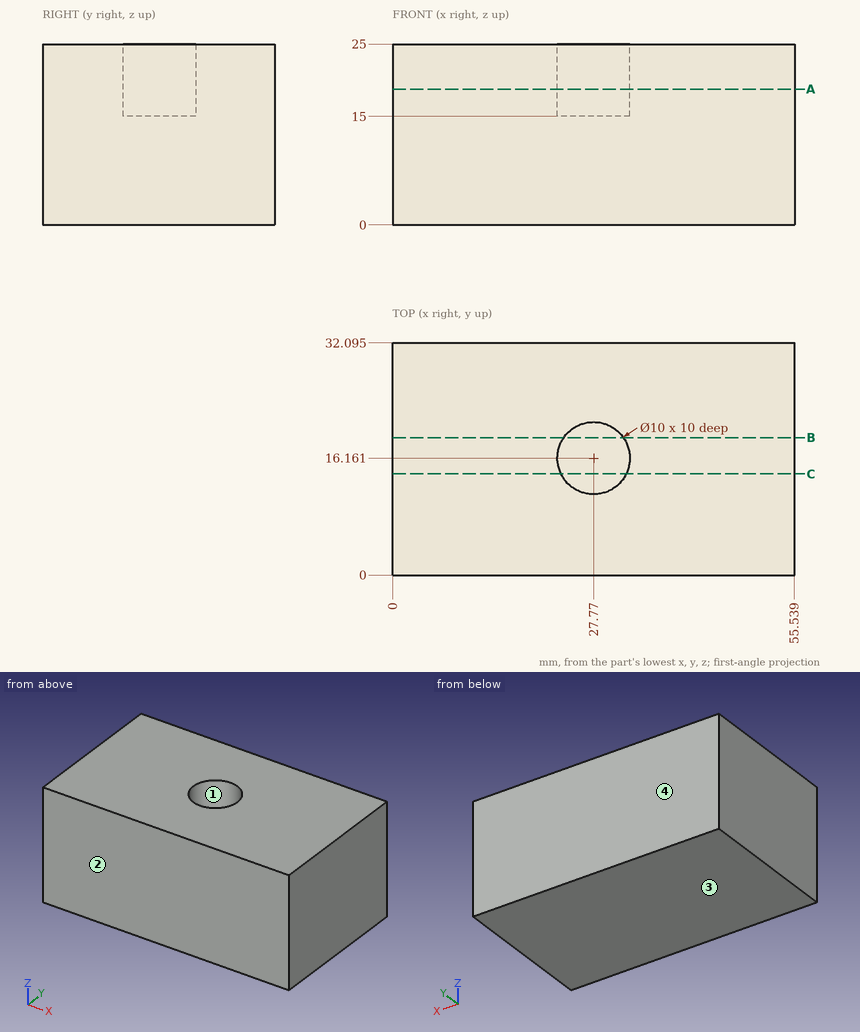
Input: dimensioned drawing with shaded views. Units: mm. Origin: part minimum x, y, z. Coordinates: 2 decimals unless noted, no trailing zeros. Order: outer loops, then holes, each group sorted by start corner. A loop starts at its lowest first (then second) coordinate and runs counter-clockwise, first axis right, second up. Notation, with made-up numbers: (9.25, 15.25) - (43.25, 15.25) arc R35 cw to (43.25, 52.25) - close; hole circle Ø5 at (-22.5, 1.25). An arc over 180 degrees is marked (long way). Return JSON: item names as keys, results as strings. Group by question number.
1. Material intervals for line 1 along Z through (x, y) = (27, 16); line 2 along X through (y, z) = (12, 17.25) (1 decimal), sorted ascending. Write a range as [from, to].
2. Cut plane B-B (y = 19). Output: boundary loops of the cut face in (x, z) (1 decimal), plus the area to 3 significant figures.
3. Cut plane C-C (y = 14). Output: boundary loops of the cut face in (x, z).
4. Pull-direction query (Y, two-part tool) for the marked faces 1, 2, 3 and 4; classes: pulls with the +Y half, pulls with the -Y half, needs draft (parallel to the pull), parting line crosses it, or undercut.
5. Cut plane A-A (z = 18.75). Output: boundary loops of the cut face in (x, y) (1 decimal), plus the area to 3 significant figures.
Resolved:
{
 "1": {"line 1": "z = [0, 15]", "line 2": "x = [0, 25], [30.5, 55.5]"},
 "2": {"outline": "(0, 0) - (55.5, 0) - (55.5, 25) - (31.9, 25) - (31.9, 15) - (23.7, 15) - (23.7, 25) - (0, 25) - close", "area": "1,310 mm²"},
 "3": {"outline": "(0, 0) - (55.54, 0) - (55.54, 25) - (32.28, 25) - (32.28, 15) - (23.26, 15) - (23.26, 25) - (0, 25) - close"},
 "4": {"face 1": "undercut", "face 2": "pulls with the -Y half", "face 3": "needs draft", "face 4": "pulls with the +Y half"},
 "5": {"outline": "(0, 0) - (55.5, 0) - (55.5, 32.1) - (0, 32.1) - close; hole circle Ø10 at (27.8, 16.2)", "area": "1,700 mm²"}
}
